from build123d import *

# Parameters (mm, degrees)
F1_DEPTH = 45
F2_R     = 8
F2_R_2   = 2.5
F3_DEPTH = 10


with BuildPart() as f1:
    # F0 (on Front) → F1 (new body)
    with BuildSketch(Plane.XZ):
        with BuildLine():
            ThreePointArc((-10, 18.483315), (-10.5, 3.5), (-11, 18.483315))
            Line((-11, 18.483315), (-11, 21.488088))
            ThreePointArc((-11, 21.488088), (-18.099342, 18.245688), (-21, 11))
            Line((-21, 11), (-21, 0))
            Line((-21, 0), (45, 0))
            Line((45, 0), (45, 3))
            Line((45, 3), (0, 3))
            Line((0, 3), (0, 11))
            ThreePointArc((0, 11), (-2.900658, 18.245688), (-10, 21.488088))
            Line((-10, 21.488088), (-10, 18.483315))
        make_face()
    extrude(amount=-F1_DEPTH)

    # F2 (on Top) → F3 (cut)
    with BuildSketch(Plane.XY):
        with Locations((22.5, 22.5)):
            Circle(F2_R)
        with Locations((6, 39)):
            Circle(F2_R_2)
        with Locations((39, 39)):
            Circle(F2_R_2)
        with Locations((39, 6)):
            Circle(F2_R_2)
        with Locations((6, 6)):
            Circle(F2_R_2)
    extrude(amount=F3_DEPTH, mode=Mode.SUBTRACT)


solid = f1.part
Work out the finished part from the listing and answer in its coordinate system (mm). A direction names the side the tool comes from. Coordinates: 2 decimals unless noted, no trailing zeros. Loops run counter-clockwise (first coordinate to the right, second up) from the corner with the lowest first, then second, coordinate; pieces in that order, holes last. Notation, with made-up numbers: (87.5, 19) -> (104.5, 19) arc R32 cw to (104.5, 51) -> close; hole circle Ø11 at (72, -6.75). An arc over 180 degrees is marked (long way). Write each question's results on one line, items separated by ' | '. Start each with the question number.
1) Consider line 1 along Y through (x, z) = (39, 2); line 2 along X through (y, z) = (39, 2.3); line 3 along Y through (x, z) = (23, 2.5). Determine where each line is inside the solid, lowest interval first.
2) The mould has two halves that part along X. Classify faces 1 (the flat face through (0, 22, 7)), 2 (the flat face through (12, 22, 0)), 3 (the cylindrical face through (16.6, 27.9, 1.5)), 4 (the flat face through (-21, 22, 6)): pulls with the +X half, pulls with the -X half, needs draft (parallel to the pull), parting line crosses it, or undercut.
3) Find section D-D on y = 6. Determine the outline of the cut face in (x, z), then the cut area to 3 significant figures.
4) Flat-ended cylindrical pins translate along their axes: P1, Ø13.5, axis at x = 28.5, y = 28.5, coming from the +Z side; P2, Ø5, axis at y = 19.5, z = 7, coming from the +X side; P3, Ø3.5, axis at y = 17.5, z = 20.5, coming from the +X side. Find the tip coordinate at first contact, or state that the pin passes through.
5) Find section B-B on x = 22.5. Determine the outline of the cut face in (y, z), then the cut area to 3 significant figures.
6) For faces 5 (the flat face through (-11, 22, 20)), 6 (the flat face through (23, 32, 3)), 7 (the flat face through (-0.4, 45, 5.2)), determine the directions among +Z, -Z, +X, -X, +Y, -Y from which every point of the face is accessible in a straight line to the end or side of a thin tool.
7) Find section C-C on y = 22.5. Determine the outline of the cut face in (x, z), then the cut area to 3 significant figures.
8) Find section A-A on x = 39. Determine the outline of the cut face in (y, z).
Response values:
1) line 1: y = 0 to 3.5, 8.5 to 36.5, 41.5 to 45 | line 2: x = -21 to 3.5, 8.5 to 36.5, 41.5 to 45 | line 3: y = 0 to 14.52, 30.48 to 45
2) face 1: pulls with the +X half | face 2: needs draft | face 3: undercut | face 4: pulls with the -X half
3) outline: (-21, 0) -> (3.5, 0) -> (3.5, 3) -> (0, 3) -> (0, 11) arc R10.5 ccw to (-10, 21.49) -> (-10, 18.48) arc R7.5 cw (long way) to (-11, 18.48) -> (-11, 21.49) arc R10.5 ccw to (-21, 11) -> close; (8.5, 0) -> (36.5, 0) -> (36.5, 3) -> (8.5, 3) -> close; (41.5, 0) -> (45, 0) -> (45, 3) -> (41.5, 3) -> close | area: 329 mm^2
4) P1: stops at z = 3 | P2: stops at x = 0 | P3: stops at x = -3.42
5) outline: (0, 0) -> (14.5, 0) -> (14.5, 3) -> (0, 3) -> close; (30.5, 0) -> (45, 0) -> (45, 3) -> (30.5, 3) -> close | area: 87.0 mm^2
6) face 5: +Z, +Y, -Y | face 6: +Z, +X, +Y, -Y | face 7: +Z, -Z, +X, -X, +Y
7) outline: (-21, 0) -> (14.5, 0) -> (14.5, 3) -> (0, 3) -> (0, 11) arc R10.5 ccw to (-10, 21.49) -> (-10, 18.48) arc R7.5 cw (long way) to (-11, 18.48) -> (-11, 21.49) arc R10.5 ccw to (-21, 11) -> close; (30.5, 0) -> (45, 0) -> (45, 3) -> (30.5, 3) -> close | area: 311 mm^2
8) outline: (0, 0) -> (3.5, 0) -> (3.5, 3) -> (0, 3) -> close; (8.5, 0) -> (36.5, 0) -> (36.5, 3) -> (8.5, 3) -> close; (41.5, 0) -> (45, 0) -> (45, 3) -> (41.5, 3) -> close
